Work out the finished part from the listing and answer in its coordinate system (mm). A direction names the side the tool comes from. Coordinates: 2 decimals unless noted, no trailing zeros. Loops run counter-clockwise (first coordinate to the right, second up) from the corner with the lowest first, then second, coordinate; pieces in that order, holes last. Notation, with made-up numbers: M 78.5,24 L 133.5,24 A13 cw 133.5,49 Z; hole C 61,-8 d5. An arc over 180 degrees is marked long. Write each question's results on one line, items separated by ' | '.
Autodesk Inventor part; units mm, degrees
ref_plane "YZ Plane" through (0, 0, 0) normal (1, 0, 0) x (0, 1, 0)
ref_plane "XZ Plane" through (0, 0, 0) normal (0, 1, 0) x (-1, 0, 0)
ref_plane "XY Plane" through (0, 0, 0) normal (0, 0, 1) x (1, 0, 0)
sketch "Esboço1" plane through (0, 0, 0) normal (1, 0, 0) x (0, 1, 0)
  line L0 (-131, 131) -> (131, 131)
  line L1 (131, 131) -> (131, -131)
  line L2 (131, -131) -> (-131, -131)
  line L3 (-131, -131) -> (-131, 131)
  line L4 (-131, 131) -> (131, -131) construction
  line L5 (131, 131) -> (-131, -131) construction
  line L6 (-15, 9) -> (15, 9)
  line L7 (15, 9) -> (15, -9)
  line L8 (15, -9) -> (-15, -9)
  line L9 (-15, -9) -> (-15, 9)
  line L10 (-15, 9) -> (15, -9) construction
  line L11 (15, 9) -> (-15, -9) construction
  point P0 (0, 0)
  dimension "d0" = 262
  dimension "d1" = 262
  dimension "d35" = 30
  dimension "d36" = 18
extrude "Extrusão1" add sketch "Esboço1" along normal mid plane 6 contours L0 L1 L2 L3 | L6 L7 L8 L9
sketch "Esboço2" plane through (3, 0, 0) normal (1, 0, 0) x (0, 0, -1)
  line L0 (131, 131) -> (-131, 131)
  line L1 (-131, 131) -> (-41.5, 131)
  line L2 (-41.5, 131) -> (-41.5, 125)
  line L3 (-41.5, 125) -> (-131, 125)
  line L4 (-131, 125) -> (-131, 131)
  line L5 (131, 131) -> (41.5, 131)
  line L6 (41.5, 131) -> (41.5, 125)
  line L7 (41.5, 125) -> (131, 125)
  line L8 (131, 125) -> (131, 131)
  line L9 (-131, 131) -> (-131, -131)
  line L10 (-131, -131) -> (-41.5, -131)
  line L11 (-41.5, -131) -> (-41.5, -125)
  line L12 (-41.5, -125) -> (-131, -125)
  line L13 (-131, -125) -> (-131, -131)
  line L14 (131, -131) -> (131, 131)
  line L15 (131, -131) -> (41.5, -131)
  line L16 (41.5, -131) -> (41.5, -125)
  line L17 (41.5, -125) -> (131, -125)
  line L18 (131, -125) -> (131, -131)
  point P0 (0, 0)
  point P1 (131, -125)
  point P2 (-131, -125)
  point P3 (41.5, 131)
  dimension "d4" = 89.5
  dimension "d5" = 6
  dimension "d6" = 89.5
  dimension "d7" = 6
  dimension "d8" = 83
  dimension "d9" = 89.5
  dimension "d10" = 6
  dimension "d11" = 89.5
  dimension "d12" = 6
  dimension "d13" = 83
extrude "Extrusão2" cut sketch "Esboço2" along normal through all both and the other way through all
sketch "Esboço3" plane through (3, 0, 0) normal (1, 0, 0) x (0, 0, -1)
  line L0 (-125, 41.5) -> (-137, 41.5)
  line L1 (-137, 41.5) -> (-137, -41.5)
  line L2 (-137, -41.5) -> (-125, -41.5)
  line L3 (-125, -41.5) -> (-125, 41.5)
  line L4 (-131, -125) -> (-131, 125)
  line L5 (-125, 41.5) -> (-137, -41.5) construction
  line L6 (-137, 41.5) -> (-125, -41.5) construction
  line L7 (125, -41.5) -> (137, -41.5)
  line L8 (137, -41.5) -> (137, 41.5)
  line L9 (137, 41.5) -> (125, 41.5)
  line L10 (125, 41.5) -> (125, -41.5)
  line L11 (131, 125) -> (131, -125)
  line L12 (125, -41.5) -> (137, 41.5) construction
  line L13 (137, -41.5) -> (125, 41.5) construction
  line L14 (-41.5, 125) -> (-131, 125)
  line L15 (-131, -125) -> (-41.5, -125)
  line L16 (131, 125) -> (41.5, 125)
  line L17 (41.5, -125) -> (131, -125)
  point P0 (0, 0)
  point P1 (-131, 0)
  point P2 (131, 0)
  dimension "d16" = 83
  dimension "d17" = 12
  dimension "d18" = 12
  dimension "d19" = 83
  dimension "d20" = 83.5
  dimension "d21" = 83.5
  dimension "d22" = 83.5
  dimension "d23" = 83.5
extrude "Extrusão3" cut sketch "Esboço3" along normal through all both and the other way through all
sketch "Esboço7" plane through (3, 0, 0) normal (1, 0, 0) x (0, 0, -1)
  line L0 (-9, 21) -> (9, 21)
  line L1 (9, 21) -> (9, -21)
  line L2 (9, -21) -> (-9, -21)
  line L3 (-9, -21) -> (-9, 21)
  line L4 (-9, 21) -> (9, -21) construction
  line L5 (9, 21) -> (-9, -21) construction
  point P0 (0, 0)
  dimension "d37" = 18
  dimension "d38" = 42
extrude "Extrusão6" cut sketch "Esboço7" against normal through all
sketch "Esboço11" plane through (3, 0, 0) normal (1, 0, 0) x (0, 0, -1)
  line L0 (-17, 0) -> (-14, 0)
  line L1 (-14, 0) -> (-14, 14)
  line L2 (-14, 14) -> (-17, 14)
  line L3 (-17, 14) -> (-17, 0)
  line L4 (-9, -21) -> (-9, 21)
  line L5 (-17, 28) -> (-14, 28)
  line L6 (-14, 28) -> (-14, 42)
  line L7 (-14, 42) -> (-17, 42)
  line L8 (-17, 42) -> (-17, 28)
  point P0 (0, 0)
  dimension "d41" = 3
  dimension "d42" = 8
  dimension "d43" = 14
  dimension "d44" = 14
  dimension "d45" = 3
  dimension "d46" = 8
  dimension "d47" = 14
  dimension "d48" = 14
extrude "Extrusão7" cut sketch "Esboço11" against normal through all
properties part number "TOPO DO POÇO 6 mm (fixed)"
1) Find section B-B, the plane x = -1.05. Give the number of separate pieces and of enclosed holes in the cut face, and give its area (3 significant figures).
Check result:
separate pieces: 1 | enclosed holes: 3 | area: 64,700 mm^2
2) Find section A-A, the plane y = 18. Give the vertices of the cut face in (x, z), and give its area (3 significant figures).
Check result:
outline: M -3,-125 L 3,-125 L 3,-9 L -3,-9 Z; M -3,9 L 3,9 L 3,125 L -3,125 Z | area: 1,390 mm^2
3) Which of the six approach directions +Z, -Z, +X, -X, +Y, -Y give full straight-line access (tool end or side, diameter ignored) to faces 1 (the face through (0, -21, 0)), 2 (the face through (0, 41.5, 128)), 3 (the face through (0, -125, 86))?
Check result:
face 1: +X, -X | face 2: +Z, +X, -X | face 3: +Z, +X, -X, -Y
4) Given pin 1 Ø1.5 at (x, z) = (0.5, -103.5) entering from +Y; pin 2 Ø1 at (x, z) = (-0.5, -97) entering from -Y; pin 3 Ø1.8 at (x, y) = (1, 128) entering from -Z, each flat-ended and moving along its own axis, determine where each tip first touches the part or whether it passes through.
Check result:
pin 1: y = 125 | pin 2: y = -125 | pin 3: z = -41.5
5) Straight lines are drawn through the part: probe 1 along Z at (x, y) = (-2.1, 4.5); probe 2 along Z at (x, y) = (-2.15, -6); probe 3 along Z at (x, y) = (-1.5, 30). For each, find the intervals that lie inside material, in ascending order. Write a range as [from, to].
Check result:
probe 1: [-125, -9], [9, 14], [17, 125] | probe 2: [-125, -9], [9, 125] | probe 3: [-125, 14], [17, 125]
6) For a pull along Y with two mould halves and no side action, classify faces 4 (the face through (0, 125, 86)), 5 (the face through (0, 41.5, -128)), 6 (the face through (0, 128, 41.5)) as released by +Y, released by -Y, zero draft, split by the parting line, or undercut.
Check result:
face 4: released by +Y | face 5: undercut | face 6: zero draft
7) Find section C-C, the plane z = 80.5. Give the vertices of the cut face in (x, y).
Check result:
outline: M -3,-125 L 3,-125 L 3,125 L -3,125 Z
